Can you work these out from the model? Positions are in its coordinate system, mm. A direction names the side the tool comes from. Round coordinates to 2 decimals unless told otherwise and drop trailing zeros. Loops run counter-clockwise (first coordinate to the right, second up) from the corner with the lowest first, then second, coordinate; pieces in that order, holes last.
(1) If I drill on line 1 along Y through (x, z) = (105, 6.35); line 2 along Y through (x, z) = (70.5, 18); line 3 along Z through (x, y) = (-103, 95), over which ranges is the centre line in solid material (lowest first)?
(2) I want a section at A-A on x = 34. Write out the boundary of the cut face in (y, z).
(3) Thinking about a two-plate mould opening in Z: for faces 4 (the face through (-9, -103, 0)), 5 (the face through (-105, 44, 243.852)), 6 (the face through (-107.95, -2, 125)), 7 (the face through (-104.731, 79.353, 6.764)), which applies, released by +Z, released by -Z, zero draft, split by the parting line, or undercut?
(4) Which directions (+Z, -Z, +X, -X, +Y, -Y) give clear straight access to the entire face, cutting with the end or side of a thin tool? Please do faces 1 (the face through (-101.6, -1, 125)), 2 (the face through (-105, 44, 247.65)), 3 (the face through (56.74, -104.73, 238.15)).
(5) I want a section at C-C on z = 121. Write out the boundary of the cut face in (x, y), plus the area to 3 significant figures.
(6) I want a section at D-D on y = 76.2. Write out the boundary of the cut face in (x, z), plus the area to 3 significant figures.
from build123d import *

# Parameters (mm, degrees)
SKETCH1_W           = 215.9
SKETCH1_H           = 215.9
SKETCH1_W_2         = 203.2
SKETCH1_H_2         = 203.2
BOSS_EXTRUDE1_DEPTH = 254
SKETCH2_W           = 25.4
SKETCH2_H           = 25.4
CUT_EXTRUDE1_DEPTH  = 216.9
SKETCH5_R           = 3.175
CUT_EXTRUDE4_DEPTH  = 6.35
SKETCH6_R           = 3.180077948
CUT_EXTRUDE5_DEPTH  = 216.9
SKETCH7_R           = 3.175
CUT_EXTRUDE6_DEPTH  = 12.7


with BuildPart() as part:
    # Sketch1 → Boss-Extrude1 (new body)
    with BuildSketch(Plane.XY):
        Rectangle(SKETCH1_W, SKETCH1_H)
        Rectangle(SKETCH1_W_2, SKETCH1_H_2, mode=Mode.SUBTRACT)
    extrude(amount=BOSS_EXTRUDE1_DEPTH)

    # Sketch2 → Cut-Extrude1 (cut, through all)
    with BuildSketch(Plane(origin=(107.95, 0, 0), x_dir=(0, 0, -1), z_dir=(1, 0, 0))):
        with Locations((-227.976799094, 53.34)):
            Rectangle(SKETCH2_W, SKETCH2_H)
        with Locations((-199.401799094, 53.34)):
            Rectangle(SKETCH2_W, SKETCH2_H)
        with BuildLine():
            Line((-243.851799094, 50.053361626), (-243.851799094, 38.064561626))
            ThreePointArc((-243.851799094, 38.064561626), (-245.750899547, 36.165461173), (-247.65, 38.064561626))
            Line((-247.65, 38.064561626), (-247.65, 50.053361626))
            ThreePointArc((-247.65, 50.053361626), (-245.750899547, 51.952462079), (-243.851799094, 50.053361626))
        make_face()
        with BuildLine():
            Line((-247.65, 56.682761626), (-247.65, 63.287106941))
            ThreePointArc((-247.65, 63.287106941), (-245.750899547, 65.186207394), (-243.851799094, 63.287106941))
            Line((-243.851799094, 63.287106941), (-243.851799094, 56.682761626))
            ThreePointArc((-243.851799094, 56.682761626), (-245.750899547, 54.783661173), (-247.65, 56.682761626))
        make_face()
        with BuildLine():
            Line((-179.728598189, 50.053361626), (-179.728598189, 38.064561626))
            ThreePointArc((-179.728598189, 38.064561626), (-181.627698642, 36.165461173), (-183.526799094, 38.064561626))
            Line((-183.526799094, 38.064561626), (-183.526799094, 50.053361626))
            ThreePointArc((-183.526799094, 50.053361626), (-181.627698642, 51.952462079), (-179.728598189, 50.053361626))
        make_face()
        with BuildLine():
            Line((-183.405698642, 56.682761626), (-183.405698642, 63.287106941))
            ThreePointArc((-183.405698642, 63.287106941), (-181.627698642, 65.065106941), (-179.849698642, 63.287106941))
            Line((-179.849698642, 63.287106941), (-179.849698642, 56.682761626))
            ThreePointArc((-179.849698642, 56.682761626), (-181.627698642, 54.904761626), (-183.405698642, 56.682761626))
        make_face()
    extrude(amount=-CUT_EXTRUDE1_DEPTH, mode=Mode.SUBTRACT)

    # Sketch5 → Cut-Extrude4 (cut)
    with BuildSketch(Plane.XZ.offset(107.95)):
        with Locations((-76.2, 6.35)):
            Circle(SKETCH5_R)
        with Locations((-50.8, 6.35)):
            Circle(SKETCH5_R)
        with Locations((0, 6.35)):
            Circle(SKETCH5_R)
        with Locations((25.4, 6.35)):
            Circle(SKETCH5_R)
    extrude(amount=-CUT_EXTRUDE4_DEPTH, mode=Mode.SUBTRACT)

    # Sketch6 → Cut-Extrude5 (cut, through all)
    with BuildSketch(Plane(origin=(107.95, 0, 0), x_dir=(0, 0, -1), z_dir=(1, 0, 0))):
        with Locations((-6.35, 95.25)):
            Circle(SKETCH6_R)
        with Locations((-6.35, 76.2)):
            Circle(SKETCH6_R)
        with Locations((-6.35, -25.4)):
            Circle(SKETCH6_R)
        with Locations((-6.35, -50.8)):
            Circle(SKETCH6_R)
        with Locations((-6.35, -76.2)):
            Circle(SKETCH6_R)
    extrude(amount=-CUT_EXTRUDE5_DEPTH, mode=Mode.SUBTRACT)

    # Sketch7 → Cut-Extrude6 (cut)
    with BuildSketch(Plane(origin=(0, -101.6, 0), x_dir=(1, 0, 0), z_dir=(0, 1, 0))):
        with Locations((-57.15, -241.3)):
            Circle(SKETCH7_R)
        with Locations((57.15, -241.3)):
            Circle(SKETCH7_R)
    extrude(amount=-CUT_EXTRUDE6_DEPTH, mode=Mode.SUBTRACT)


solid = part.part
Filled sheet:
1. line 1: y = -107.95 to -79.38, -73.02 to -53.98, -47.62 to -28.58, -22.22 to 73.02, 79.38 to 92.07, 98.43 to 107.95
1. line 2: y = -107.95 to -101.6, 101.6 to 107.95
1. line 3: z = 0 to 3.18, 9.52 to 254
2. outline: (-107.95, 0) - (-101.6, 0) - (-101.6, 254) - (-107.95, 254) - close; (101.6, 0) - (107.95, 0) - (107.95, 254) - (101.6, 254) - close
3. face 4: released by -Z
3. face 5: undercut
3. face 6: zero draft
3. face 7: undercut
4. face 1: +Z, -Z
4. face 2: +X, -X
4. face 3: -Y
5. outline: (-107.95, -107.95) - (107.95, -107.95) - (107.95, 107.95) - (-107.95, 107.95) - close; hole (-101.6, -101.6) - (101.6, -101.6) - (101.6, 101.6) - (-101.6, 101.6) - close
5. area: 5,320 mm2
6. outline: (-107.95, 0) - (-101.6, 0) - (-101.6, 3.17) - (-107.95, 3.17) - close; (-107.95, 9.53) - (-101.6, 9.53) - (-101.6, 254) - (-107.95, 254) - close; (101.6, 0) - (107.95, 0) - (107.95, 3.17) - (101.6, 3.17) - close; (101.6, 9.53) - (107.95, 9.53) - (107.95, 254) - (101.6, 254) - close
6. area: 3,150 mm2
